```python
from build123d import *

# Parameters (mm, degrees)
SKETCH_1_W      = 30
SKETCH_1_H      = 35
SKETCH_1_R      = 1.6
EXTRUDE_1_DEPTH = 2
SKETCH_2_W      = 9
SKETCH_2_H      = 8
EXTRUDE_2_DEPTH = 3.2
SKETCH_3_W      = 3.8
SKETCH_3_H      = 6
EXTRUDE_3_DEPTH = 4.5
SKETCH_4_W      = 14
SKETCH_4_H      = 6
EXTRUDE_4_DEPTH = 1.5
FILLET_1_R      = 1.6
FILLET_2_R      = 2
SKETCH_5_W      = 4
SKETCH_5_H      = 4.2
EXTRUDE_5_DEPTH = 4
EXTRUDE_6_DEPTH = 10


with BuildPart() as part:
    # 草图1 → 凸台-拉伸1 (new body)
    with BuildSketch(Plane.XY):
        with Locations((15, 17.5)):
            Rectangle(SKETCH_1_W, SKETCH_1_H)
        with Locations((5, 32)):
            Circle(SKETCH_1_R, mode=Mode.SUBTRACT)
        with Locations((25, 32)):
            Circle(SKETCH_1_R, mode=Mode.SUBTRACT)
        with Locations((5, 3.3)):
            Circle(SKETCH_1_R, mode=Mode.SUBTRACT)
        with Locations((25, 3.3)):
            Circle(SKETCH_1_R, mode=Mode.SUBTRACT)
    extrude(amount=EXTRUDE_1_DEPTH)

    # 草图2 → 凸台-拉伸2 (add)
    with BuildSketch(Plane.XY.offset(2)):
        with Locations((15, 3)):
            Rectangle(SKETCH_2_W, SKETCH_2_H)
    extrude(amount=EXTRUDE_2_DEPTH)

    # 草图3 → 凸台-拉伸3 (add)
    with BuildSketch(Plane.XY.offset(2)):
        with Locations((2.1, 10)):
            Rectangle(SKETCH_3_W, SKETCH_3_H)
        with Locations((27.9, 10)):
            Rectangle(SKETCH_3_W, SKETCH_3_H)
    extrude(amount=EXTRUDE_3_DEPTH)

    # 草图4 → 凸台-拉伸4 (add)
    with BuildSketch(Plane(origin=(0, 0, 0), x_dir=(-1, 0, 0), z_dir=(0, 0, -1))):
        with Locations((-15, 3)):
            Rectangle(SKETCH_4_W, SKETCH_4_H)
    extrude(amount=EXTRUDE_4_DEPTH)

    # 圆角1
    fillet_1_edges = [part.edges().sort_by_distance(p)[0] for p in [
        (19.5, 3, 5.2),
        (19.5, -0.5, 2),
        (10.5, -0.5, 2),
        (10.5, 3, 5.2),
    ]]
    fillet(fillet_1_edges, radius=FILLET_1_R - 0.0001)  # a hair under: the kernel refuses the full size

    # 圆角2
    fillet_2_edges = [part.edges().sort_by_distance(p)[0] for p in [
        (0, 35, 1),
        (30, 35, 1),
        (30, 0, 1),
        (0, 0, 1),
    ]]
    fillet(fillet_2_edges, radius=FILLET_2_R)

    # 草图5 → 凸台-拉伸5 (add)
    with BuildSketch(Plane.ZY.offset(-0.2)):
        with Locations((4.25, 10)):
            Rectangle(SKETCH_5_W, SKETCH_5_H)
    extrude_5 = extrude(amount=EXTRUDE_5_DEPTH)

    # 镜向1: 凸台-拉伸5 across plane
    add(extrude_5.mirror(Plane.ZY.offset(-15)))

    # 草图6 → 凸台-拉伸6 (add)
    with BuildSketch(Plane.XZ.offset(1)):
        with BuildLine():
            Line((17.5, 0.6), (12.5, 0.6))
            ThreePointArc((12.5, 0.6), (9.5, 3.6), (12.5, 6.6))
            Line((12.5, 6.6), (17.5, 6.6))
            ThreePointArc((17.5, 6.6), (20.5, 3.6), (17.5, 0.6))
        make_face()
    extrude(amount=EXTRUDE_6_DEPTH)


solid = part.part
```
Check sheet for the modelled part. Datum: model origin and axes. Units: mm. A direction names the side the tool comes from. Round coordinates to 2 decimals unless told otherwise and drop trailing zeros. Loops run counter-clockwise (first coordinate to the right, second up) from the corner with the lowest first, then second, coordinate; pieces in that order, holes last. Notation, with made-up numbers: (0.25, -9.75) - (6.25, -9.75) arc R32 cw to (6.25, 17.25) - close; hole circle Ø6 at (-38.75, 32). An arc over 180 degrees is marked (long way). Write item = value, one per line. Start each with the question number.
Q1. Depth check by flat-ended pin: P1, Ø4.5, axis at x = 32.5, z = 4, coming from the +Y side; P2, Ø3, axis at x = 4.5, y = 3, coming from the +Z side; P3, Ø2, axis at x = 9, z = 4, coming from the +Y side. Enter the tip coordinate at first touch or a pass-through.
Q2. Section check B-B (z = 4.5). Record the boundary of the cut face in (x, y).
Q3. Section check A-A (x = 5). Record the boundary of the cut face in (y, z), plus the area to 3 significant figures.
Q4. Access from +Z, -Z, +X, -X, +Y, -Y to the whole of each face (thin tool, end or side, straight path). Record for faces 1 (the face through (15, -6, 0.6)), 2 (the face through (15, -1, 6)), 3 (the face through (10.96, -0.49, 2.48)), 4 (the face through (4, 10, 4)).
Q5. Thickness scan on L1, parallel to Y at x = 5, z = 1.3; L2, parallel to Y at x = 15, z = 1.5; L3, parallel to Z at x = 14.5, y = 23.5. Record the ranges inside material, lowest first.
Q6. Section check D-D (z = 1.5). Record the boundary of the cut face in (x, y).
Q7. Release check for a two-part mould opening along X. For faces 5 (the face through (0.57, 34.4, 1.01)), 6 (the face through (23.82, 4.38, 0.99)), 7 (the face through (15, -0.5, 2)) record: pulls with the +X half, pulls with the -X half, needs draft (parallel to the pull), parting line crosses it, or undercut.
Q8. Section check C-C (y = 32). Record the boundary of the cut face in (x, z).
Derived:
q1.P1 = 12.1
q1.P2 = 2
q1.P3 = -1
q2.outline = (-3.8, 7.9) - (0.2, 7.9) - (0.2, 7) - (4, 7) - (4, 13) - (0.2, 13) - (0.2, 12.1) - (-3.8, 12.1) - close; (9.64, -11) - (20.36, -11) - (20.36, -1) - (19.22, -1) - (19.22, 7) - (10.78, 7) - (10.78, -1) - (9.64, -1) - close; (26, 7) - (29.8, 7) - (29.8, 7.9) - (33.8, 7.9) - (33.8, 12.1) - (29.8, 12.1) - (29.8, 13) - (26, 13) - close
q3.outline = (0, 0) - (1.7, 0) - (1.7, 2) - (0, 2) - close; (4.9, 0) - (30.4, 0) - (30.4, 2) - (4.9, 2) - close; (33.6, 0) - (35, 0) - (35, 2) - (33.6, 2) - close
q3.area = 57.2 mm^2
q4.face_1 = -Z, +X, -X, -Y
q4.face_2 = none
q4.face_3 = -Z, -X
q4.face_4 = +Z, +Y, -Y
q5.L1 = 0 to 1.7, 4.9 to 30.4, 33.6 to 35
q5.L2 = -11 to -1, 0 to 35
q5.L3 = 0 to 2
q6.outline = (0, 2) arc R2 ccw to (2, 0) - (28, 0) arc R2 ccw to (30, 2) - (30, 33) arc R2 ccw to (28, 35) - (2, 35) arc R2 ccw to (0, 33) - close; (10.36, -11) - (19.64, -11) - (19.64, -1) - (10.36, -1) - close; hole circle Ø3.2 at (5, 3.3); hole circle Ø3.2 at (5, 32); hole circle Ø3.2 at (25, 3.3); hole circle Ø3.2 at (25, 32)
q7.face_5 = pulls with the -X half
q7.face_6 = undercut
q7.face_7 = needs draft
q8.outline = (0, 0) - (3.4, 0) - (3.4, 2) - (0, 2) - close; (6.6, 0) - (23.4, 0) - (23.4, 2) - (6.6, 2) - close; (26.6, 0) - (30, 0) - (30, 2) - (26.6, 2) - close
